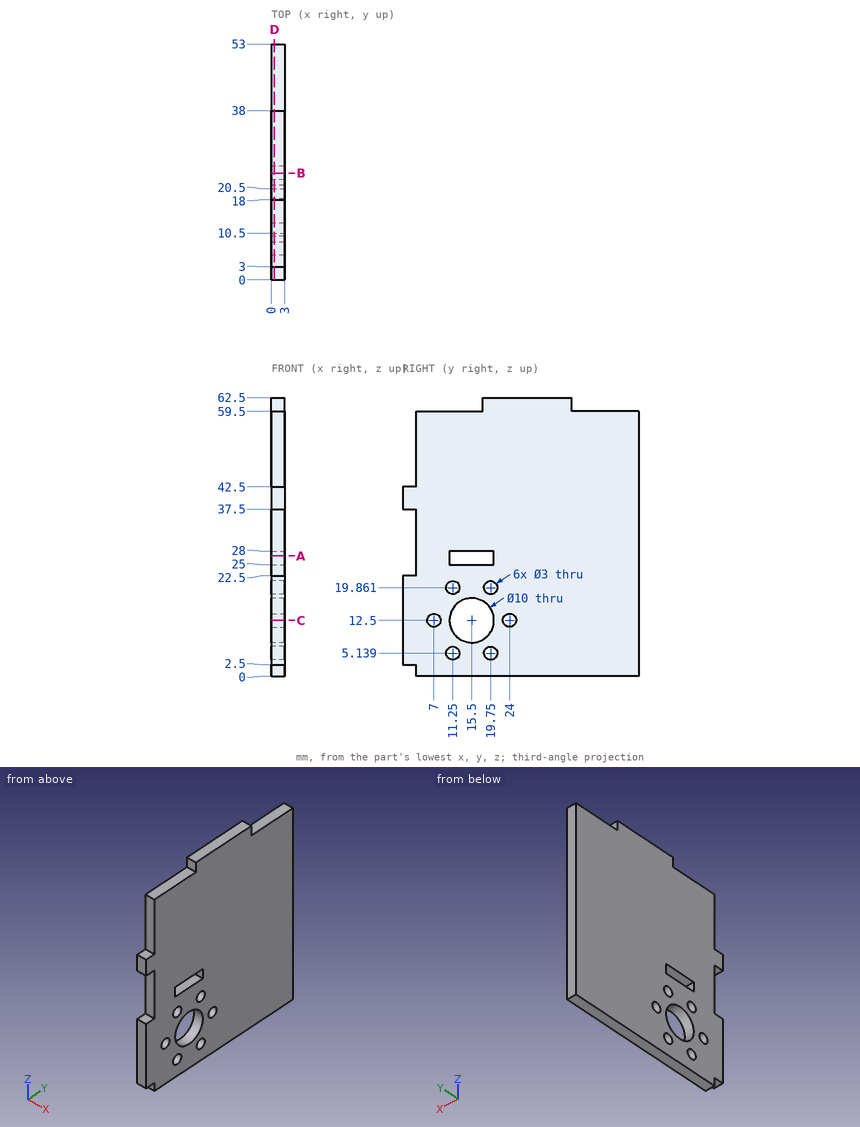
Job drawing, mm, ordinate dimensions from the low corner. One solid piece. Round coordinates to 2 decimals unless told otherwise and drop trailing zeros. Order: outer loops, then holes, each group sorted by start corner. A loop starts at its lowest first (then second) coordinate and runs counter-clockwise, first axis right, second up. Notation, with made-up numbers: (32, 65.25) -> (37, 65.25) arc R28 ccw to (37, 91.25) -> close; hole circle Ø4 at (69.25, -25.5). An arc over 180 degrees is marked (long way). Answer in a Markdown table with one row per item.
1) Band-saw the part on D-D on x = 0.65. Give the number of separate pieces and of enclosed holes in the cut face, and give its area (3 significant figures).
Values:
| item | result |
|---|---|
| separate pieces | 1 |
| enclosed holes | 8 |
| area | 2,960 mm2 |
2) Band-saw the part on C-C on z = 12.5. Give the cut face in (x, y).
Values:
| item | result |
|---|---|
| outline | (0, 0) -> (3, 0) -> (3, 5.5) -> (0, 5.5) -> close; (0, 8.5) -> (3, 8.5) -> (3, 10.5) -> (0, 10.5) -> close; (0, 20.5) -> (3, 20.5) -> (3, 22.5) -> (0, 22.5) -> close; (0, 25.5) -> (3, 25.5) -> (3, 53) -> (0, 53) -> close |
3) Wall check: L1, parallel to Z at x = 0.8, y = 43.5; L2, parallel to Y at x = 1.05, z = 18.5; L3, parallel to Z at x = 2.35, y = 7. Give the ranges that are in metal, low to high.
Values:
| item | result |
|---|---|
| L1 | 0 to 59.5 |
| L2 | 0 to 10.62, 11.88 to 19.12, 20.38 to 53 |
| L3 | 0 to 11, 14 to 59.5 |
4) Band-saw the part on A-A on z = 27. Give the cut face in (x, y), and give its area (3 significant figures).
Values:
| item | result |
|---|---|
| outline | (0, 3) -> (3, 3) -> (3, 10.5) -> (0, 10.5) -> close; (0, 20.5) -> (3, 20.5) -> (3, 53) -> (0, 53) -> close |
| area | 120 mm2 |
5) Band-saw the part on B-B on y = 24. Give the cut face in (x, z).
Values:
| item | result |
|---|---|
| outline | (0, 0) -> (3, 0) -> (3, 11) -> (0, 11) -> close; (0, 14) -> (3, 14) -> (3, 62.5) -> (0, 62.5) -> close |
6) Pin check, flat tips, straight feed: P1, Ø0.9, axis at x = 2, z = 26.5, coming from the -Y side; P2, Ø2.5, axis at y = 7, z = 12.5, coming from the +X side; P3, Ø0.9, axis at x = 1.5, y = 13.5, coming from the +Z side. Stop position of each tip, or through.
Values:
| item | result |
|---|---|
| P1 | y = 3 |
| P2 | through |
| P3 | z = 59.5 |
